```python
from build123d import *

# Parameters (mm, degrees)
BOSS_EXTRUDE1_DEPTH = 11
SKETCH2_R           = 15
BOSS_EXTRUDE2_DEPTH = 25
SKETCH5_R           = 10
CUT_EXTRUDE1_DEPTH  = 20
SKETCH8_R           = 7.5
CUT_EXTRUDE2_DEPTH  = 93.021736563
SKETCH13_R          = 7.5
CUT_EXTRUDE3_DEPTH  = 93.021736563
SKETCH14_W          = 36
SKETCH14_H          = 20
CUT_EXTRUDE4_DEPTH  = 5
SKETCH18_W          = 40.91
SKETCH18_H          = 7
BOSS_EXTRUDE5_DEPTH = 15


with BuildPart() as part:
    # Sketch1 → Boss-Extrude1 (new body)
    with BuildSketch(Plane(origin=(0, 0, 0), x_dir=(1, 0, 0), z_dir=(0, 1, 0))):
        with BuildLine():
            Line((0, 18), (70, 18))
            ThreePointArc((70, 18), (88, 0), (70, -18))
            Line((70, -18), (0, -18))
            ThreePointArc((0, -18), (-18, 0), (0, 18))
        make_face()
    extrude(amount=BOSS_EXTRUDE1_DEPTH)

    # Sketch2 → Boss-Extrude2 (add)
    with BuildSketch(Plane(origin=(0, 11, 0), x_dir=(1, 0, 0), z_dir=(0, 1, 0))):
        with Locations(Location((0, 0, 0), (0, 0, 270))):
            Circle(SKETCH2_R)
        with Locations(Location((70, 0, 0), (0, 0, 270))):
            Circle(SKETCH2_R)
    extrude(amount=BOSS_EXTRUDE2_DEPTH)

    # Sketch5 → Cut-Extrude1 (cut)
    with BuildSketch(Plane(origin=(0, 36, 0), x_dir=(1, 0, 0), z_dir=(0, 1, 0))):
        with Locations(Location((70, 0, 0), (0, 0, 270))):
            Circle(SKETCH5_R)
        with Locations(Location((0, 0, 0), (0, 0, 270))):
            Circle(SKETCH5_R)
    extrude(amount=-CUT_EXTRUDE1_DEPTH, mode=Mode.SUBTRACT)

    # Sketch8 → Cut-Extrude2 (cut, through all)
    with BuildSketch(Plane(origin=(0, 16, 0), x_dir=(1, 0, 0), z_dir=(0, 1, 0))):
        with Locations(Location((0, 0, 0), (0, 0, 270))):
            Circle(SKETCH8_R)
    extrude(amount=-CUT_EXTRUDE2_DEPTH, mode=Mode.SUBTRACT)

    # Sketch13 → Cut-Extrude3 (cut, through all)
    with BuildSketch(Plane(origin=(0, 16, 0), x_dir=(1, 0, 0), z_dir=(0, 1, 0))):
        with Locations(Location((70, 0, 0), (0, 0, 270))):
            Circle(SKETCH13_R)
    extrude(amount=-CUT_EXTRUDE3_DEPTH, mode=Mode.SUBTRACT)

    # Sketch14 → Cut-Extrude4 (cut)
    with BuildSketch(Plane.XZ):
        with Locations((34.999969462, -0.04623456)):
            Rectangle(SKETCH14_W, SKETCH14_H)
    extrude(amount=-CUT_EXTRUDE4_DEPTH, mode=Mode.SUBTRACT)

    # Sketch18 → Boss-Extrude5 (add)
    with BuildSketch(Plane(origin=(0, 11, 0), x_dir=(1, 0, 0), z_dir=(0, 1, 0))):
        with Locations((35, 0)):
            Rectangle(SKETCH18_W, SKETCH18_H)
    extrude(amount=BOSS_EXTRUDE5_DEPTH)


solid = part.part
```
Source: CAD feature listing. Evaluate the final solid. Frame: model axes, mm. A direction names the side the tool comes from. Round coordinates to 2 decimals unless told otherwise and drop trailing zeros. Order: outer loops, then holes, each group sorted by start corner. A loop starts at its lowest first (then second) coordinate and runs counter-clockwise, first axis right, second up. Notation, with made-up numbers: (5.25, 26.25) -> (58.25, 26.25) arc R22 cw to (58.25, 61.25) -> close; hole circle Ø1 at (9, 4.5). An arc over 180 degrees is marked (long way). Use CSV: the item, a comma, the result in double quotes.
(1) Access query for faces 4 (the face through (79.915, 26.14, -1.302)), 5 (the face through (35, 26, 0)), 6 (the face through (-10, 36, 3)), 7 (the face through (35, 2, 9.954)), 8 (the face through (36, 0, 12)). Directions: +Z, -Z, +X, -X, +Y, -Y. A direction counts if a zero-diameter tool reaches every point of the face in a straight line with its end or side. Return the directions, or none.
Report:
face 4,"+Y"
face 5,"+Z, -Z, +Y"
face 6,"+Z, -Z, +X, -X, +Y"
face 7,"-Y"
face 8,"+Z, -Z, +X, -X, -Y"
(2) Section D-D on y = 29. Return the cut outline in (x, z), and give its area (3 significant figures).
Report:
outline,"circle Ø30 at (0, 0); circle Ø30 at (70, 0); hole circle Ø20 at (0, 0); hole circle Ø20 at (70, 0)"
area,"785 mm^2"
(3) Pull-direction query (X, two-part tool) for faces 1 (the face through (35, 18, 3.5)), 2 (the face through (35, 5, 18)), 3 (the face through (88, 5, 0)); classes: +X half, -X half, draft (parallel to the pull), parting line (faces both ways), or undercut.
Report:
face 1,"undercut"
face 2,"draft"
face 3,"+X half"
(4) First-contact query: pin 1 Ø4 at (y, z) = (19.5, 12) entering from -X; pin 2 Ø18 at (x, z) = (70, 0) entering from +Y; pin 3 Ø2.5 at (y, z) = (3, -0.5) entering from -X; pin 4 Ø10 at (x, z) = (-4, -3.5) entering from +Y. Flat tips, straight axial feed; report the tip coordinate or a pass-through.
Report:
pin 1,"x = -11.18"
pin 2,"y = 16"
pin 3,"x = -18"
pin 4,"y = 36"
(5) Ray query, L1, parallel to X at y = 4, z = 0; L2, parallel to X at y = 31.5, z = 0; L3, parallel to X at y = 20, z = 0. Return the intervals inside material, ascending.
Report:
L1,"-18 to -7.5, 7.5 to 17, 53 to 62.5, 77.5 to 88"
L2,"-15 to -10, 10 to 15, 55 to 60, 80 to 85"
L3,"-15 to -10, 10 to 60, 80 to 85"
(6) Section C-C on x = 50. Return the cut outline in (y, z), and give its area (3 significant figures).
Report:
outline,"(0, -18) -> (11, -18) -> (11, -3.5) -> (26, -3.5) -> (26, 3.5) -> (11, 3.5) -> (11, 18) -> (0, 18) -> (0, 9.95) -> (5, 9.95) -> (5, -10.05) -> (0, -10.05) -> close"
area,"401 mm^2"
(7) Section A-A on z = 0. Count the separate pieces of the cut face and the enclosed holes in it, and give its area (3 significant figures).
Report:
separate pieces,"3"
enclosed holes,"0"
area,"1,810 mm^2"
(8) Section B-B on y = 23. Return the cut outline in (x, z), and give its area (3 significant figures).
Report:
outline,"(14.59, -3.5) -> (55.41, -3.5) arc R15 ccw (long way) to (55.41, 3.5) -> (14.59, 3.5) arc R15 ccw (long way) to start; hole circle Ø20 at (0, 0); hole circle Ø20 at (70, 0)"
area,"1,070 mm^2"
